The model under review builds one solid part; all positions refer to its coordinate system, in mm. Face numbers are marked on the shaded views. Round coordinates to 2 decimals unless told otherwise and drop trailing zeros. Loops run counter-clockwise (first coordinate to the right, second up) from the corner with the lowest first, then second, coordinate; pieces in that order, holes last. Notation, with made-up numbers: M -3.5,4.5 L 31.5,4.5 A33 ccw 31.5,34.5 Z; hole C -35.75,18 d4. An arc over 180 degrees is marked long. Return JSON: item names as keys, results as strings. Group by question number.
Q1. Consider section B-B (x = 83). State the section outline as (y, z) points, and give its area (3 significant figures).
Q2. Consider section A-A (z = -34). State the section outline as (x, y) points.
Q3. Clearance check with flat-ended pins moving along their axes: pin 1 Ø10 at (x, z) = (118.5, -74) entering from +Y; pin 2 Ø10 at (y, z) = (-29, -63.5) entering from +X; pin 3 Ø6 at (x, y) = (-147.4, -30.91) entering from +Z; pin 4 Ø8 at (x, y) = (-148, -30) entering from -Z. State where each tip first meets the part, or that it passes through.
Q4. To check wall thickness, follow line 1 along Y through (x, z) = (147.4, -2.8); line 2 along X through (y, z) = (-39.5, -92.5); line 3 along Y through (x, z) = (-33, -40.5). State the ranges of each line that lie inside material, in increasing order.
Q5. Draft analysis for pull direction X (two halves, no side actions). For the marked faces 1 and 2, state which applies: pulls with the +X half, pulls with the -X half, needs draft (parallel to the pull), parting line crosses it, or undercut.
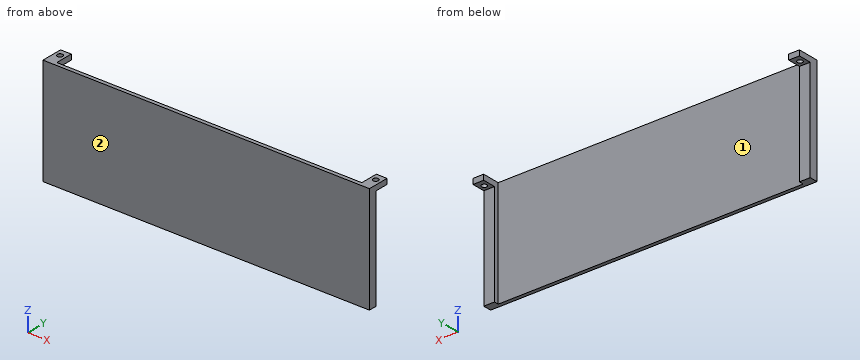
from build123d import *

# Parameters (mm, degrees)
SKETCH1_W                       = 10
SKETCH1_H                       = 16.5
BOSS_EXTRUDE1_DEPTH             = 100
F_5_0MM_DOWEL_HOLE3_D           = 5
F_5_0MM_DOWEL_HOLE3_DEPTH       = 100
F_5_0MM_DOWEL_HOLE3_CSINK_D     = 5.05
F_5_0MM_DOWEL_HOLE3_CSINK_ANGLE = 90
F_5_0MM_DOWEL_HOLE3_TIP         = 1.502151548
SKETCH8_R                       = 2.5
BOSS_EXTRUDE2_DEPTH             = 100
SKETCH11_W                      = 7.604101256
SKETCH11_H                      = 6.322975501
BOSS_EXTRUDE3_DEPTH             = 10
SKETCH10_W                      = 95
SKETCH10_H                      = 12.25
CUT_EXTRUDE3_DEPTH              = 10
SKETCH12_W                      = 7.319773992
SKETCH12_H                      = 6.84369113
BOSS_EXTRUDE4_DEPTH             = 5


with BuildPart() as part:
    # Sketch1 → Boss-Extrude1 (new body)
    with BuildSketch(Plane.XY):
        Polygon((-152.4, -40.74), (-142.4, -40.74), (-142.4, -24.24), (-152.4, -24.24), (-152.4, -24.840528939), align=None)
        Polygon((0, -44.24), (0, -40.74), (-142.4, -40.74), (-152.4, -40.74), (-152.4, -44.24), align=None)
        Polygon((142.4, -40.74), (0, -40.74), (0, -44.24), (152.4, -44.24), (152.4, -40.74), align=None)
        with Locations((147.4, -32.49)):
            Rectangle(SKETCH1_W, SKETCH1_H)
    extrude(amount=-BOSS_EXTRUDE1_DEPTH)

    # Ø5.0mm Dowel Hole3
    with Locations(Plane.XY):
        with Locations((-147.4, -30.906666667), (-147.4, -37.573333333), (147.4, -30.906666667), (147.4, -37.573333333)):
            CounterSinkHole(F_5_0MM_DOWEL_HOLE3_D / 2, F_5_0MM_DOWEL_HOLE3_CSINK_D / 2, depth=F_5_0MM_DOWEL_HOLE3_DEPTH, counter_sink_angle=F_5_0MM_DOWEL_HOLE3_CSINK_ANGLE)
            with Locations((0, 0, -(F_5_0MM_DOWEL_HOLE3_DEPTH + F_5_0MM_DOWEL_HOLE3_TIP / 2))):  # 118° drill point
                Cone(0, F_5_0MM_DOWEL_HOLE3_D / 2, F_5_0MM_DOWEL_HOLE3_TIP, mode=Mode.SUBTRACT)

    # Sketch8 → Boss-Extrude2 (add)
    with BuildSketch(Plane(origin=(0, 0, -100), x_dir=(-1, 0, 0), z_dir=(0, 0, -1))):
        with Locations((147.4, -37.573333333)):
            Circle(SKETCH8_R)
    boss_extrude2 = extrude(amount=-BOSS_EXTRUDE2_DEPTH)

    # Sketch11 → Boss-Extrude3 (add)
    with BuildSketch(Plane.XY):
        with Locations((-147.317312743, -37.707651596)):
            Rectangle(SKETCH11_W, SKETCH11_H)
    extrude(amount=-BOSS_EXTRUDE3_DEPTH)

    # Mirror4: Boss-Extrude2 across plane
    add(boss_extrude2.mirror(Plane(origin=(0, 0, 0), x_dir=(0, 0, 1), z_dir=(1, 0, 0))))

    # Sketch10 → Cut-Extrude3 (cut)
    with BuildSketch(Plane(origin=(152.4, 0, 0), x_dir=(0, 0, -1), z_dir=(1, 0, 0))):
        with Locations((52.5, -30.365)):
            Rectangle(SKETCH10_W, SKETCH10_H)
    cut_extrude3 = extrude(amount=-CUT_EXTRUDE3_DEPTH, mode=Mode.SUBTRACT)

    # Mirror5: Cut-Extrude3 across plane
    add(cut_extrude3.mirror(Plane(origin=(0, 0, 0), x_dir=(0, 0, 1), z_dir=(1, 0, 0))), mode=Mode.SUBTRACT)

    # Sketch12 → Boss-Extrude4 (add)
    with BuildSketch(Plane.XY):
        with Locations((147.557359199, -37.793735485)):
            Rectangle(SKETCH12_W, SKETCH12_H)
    extrude(amount=-BOSS_EXTRUDE4_DEPTH)


solid = part.part
Values:
{
 "1": {"outline": "M -44.24,-100 L -40.74,-100 L -40.74,0 L -44.24,0 Z", "area": "350 mm2"},
 "2": {"outline": "M -152.4,-44.24 L 152.4,-44.24 L 152.4,-36.49 L 142.4,-36.49 L 142.4,-40.74 L -142.4,-40.74 L -142.4,-36.49 L -152.4,-36.49 Z"},
 "3": {"pin 1": "stops at y = -40.74", "pin 2": "passes through", "pin 3": "stops at z = 0", "pin 4": "stops at z = -5"},
 "4": {"line 1": "y = -44.24 to -33.41, -28.41 to -24.24", "line 2": "x = -152.4 to -142.4, 142.4 to 152.4", "line 3": "y = -44.24 to -40.74"},
 "5": {"face 1": "undercut", "face 2": "needs draft"}
}
